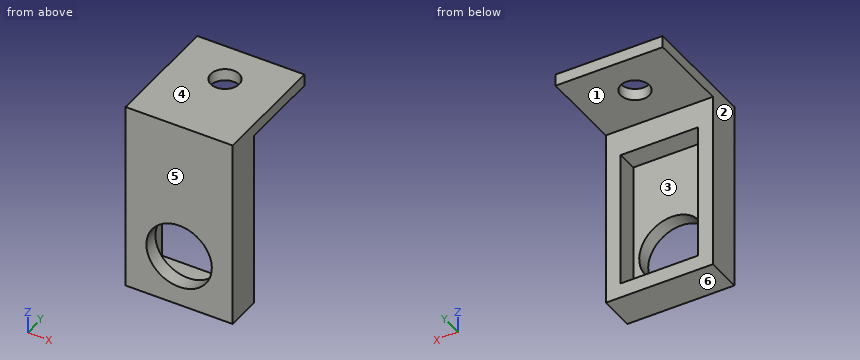
from build123d import *

# Parameters (mm, degrees)
SKETCH1_W           = 18
SKETCH1_H           = 32
BOSS_EXTRUDE1_DEPTH = 6
SKETCH2_W           = 13
SKETCH2_H           = 23
CUT_EXTRUDE1_DEPTH  = 3.5
SKETCH3_R           = 5.5
CUT_EXTRUDE2_DEPTH  = 37.881567212
SKETCH4_W           = 18
SKETCH4_H           = 2
BOSS_EXTRUDE2_DEPTH = 14
SKETCH5_R           = 2.4
CUT_EXTRUDE3_DEPTH  = 41.298883359


with BuildPart() as part:
    # Sketch1 → Boss-Extrude1 (new body)
    with BuildSketch(Plane(origin=(0, 0, 0), x_dir=(1, 0, 0), z_dir=(0, 1, 0))):
        with Locations((9, 16)):
            Rectangle(SKETCH1_W, SKETCH1_H)
    extrude(amount=BOSS_EXTRUDE1_DEPTH)

    # Sketch2 → Cut-Extrude1 (cut)
    with BuildSketch(Plane(origin=(0, 6, 0), x_dir=(1, 0, 0), z_dir=(0, 1, 0))):
        with Locations((9, 18)):
            Rectangle(SKETCH2_W, SKETCH2_H)
    extrude(amount=-CUT_EXTRUDE1_DEPTH, mode=Mode.SUBTRACT)

    # Sketch3 → Cut-Extrude2 (cut, through all)
    with BuildSketch(Plane(origin=(0, 2.5, 0), x_dir=(1, 0, 0), z_dir=(0, 1, 0))):
        with Locations(Location((9.000820155, 23.3, 0), (0, 0, 270))):
            Circle(SKETCH3_R)
    extrude(amount=-CUT_EXTRUDE2_DEPTH, mode=Mode.SUBTRACT)

    # Sketch4 → Boss-Extrude2 (add)
    with BuildSketch(Plane(origin=(0, 6, 0), x_dir=(1, 0, 0), z_dir=(0, 1, 0))):
        with Locations((9, 1)):
            Rectangle(SKETCH4_W, SKETCH4_H)
    extrude(amount=BOSS_EXTRUDE2_DEPTH)

    # Sketch5 → Cut-Extrude3 (cut, through all)
    with BuildSketch(Plane(origin=(0, 0, -2), x_dir=(-1, 0, 0), z_dir=(0, 0, -1))):
        with Locations((-8.774181154, 13.15523395)):
            Circle(SKETCH5_R)
    extrude(amount=-CUT_EXTRUDE3_DEPTH, mode=Mode.SUBTRACT)


solid = part.part
The model under review builds one solid part; all positions refer to its coordinate system, in mm. Face numbers are marked on the shaded views. A direction names the side the tool comes from. Round coordinates to 2 decimals unless told otherwise and drop trailing zeros. Write each loop counter-clockwise with the first axis right and the second up, starting at its lowest first coordinate (ties: lowest second). Pieces come first, ordered by that corner, then holes. Notation, with made-up numbers: (19.25, -18.75) - (64.25, -18.75) arc R31 cw to (64.25, 7.25) - close; hole circle Ø9 at (41, 78.25). An arc over 180 degrees is marked (long way). One line per item, written item: value. Start each with the question number.
1. Consider section D-D on z = -19. Write out the cut boundary in (x, y), and give its area (3 significant figures).
2. Consider section A-A on z = -23.3. Write out the cut boundary in (x, y).
3. Clearance check with flat-ended pins moving along their axes: P1, Ø3, axis at y = 9.5, z = -4, coming from the -X side; P2, Ø4, axis at x = 9, z = -13, coming from the +Y side; P3, Ø2, axis at x = 5, y = 13.5, coming from the -Z side. State where each tip first meets the part, or that it passes through.
4. The part is to be moulded in two halves that separate along Z. For the marked faces 3, 4, 5 and 6, say which applies: released by +Z, released by -Z, zero draft, split by the parting line, or undercut.
5. To check wall thickness, follow L1, parallel to X at y = 0.7, z = -23.3; L2, parallel to X at y = 5, z = -28; L3, parallel to Z at x = 13.75, y = 18.5. State the ranges of each line that lie inside material, in increasing order. Write a range as from..to.
6. Consider section C-C on x = 4. Write out the cut boundary in (y, z), and give its area (3 significant figures).
7. Consider section B-B on y = 4.75. Write out the cut boundary in (x, z).
8. Machinability: for the marked faces 1 and 2, which of the approach directions +Z, -Z, +X, -X, +Y, -Y give a long, thin tool a straight path to every point of the face, cutting with its end or side? Answer none if there is none.
Checks:
1. outline: (0, 0) - (5.57, 0) - (5.57, 2.5) - (2.5, 2.5) - (2.5, 6) - (0, 6) - close; (12.43, 0) - (18, 0) - (18, 6) - (15.5, 6) - (15.5, 2.5) - (12.43, 2.5) - close
1. area: 45.4 mm^2
2. outline: (0, 0) - (3.5, 0) - (3.5, 2.5) - (2.5, 2.5) - (2.5, 6) - (0, 6) - close; (14.5, 0) - (18, 0) - (18, 6) - (15.5, 6) - (15.5, 2.5) - (14.5, 2.5) - close
3. P1: passes through
3. P2: stops at y = 2.5
3. P3: stops at z = -2
4. face 3: undercut
4. face 4: released by +Z
4. face 5: zero draft
4. face 6: released by -Z
5. L1: x = 0..3.5, 14.5..18
5. L2: x = 0..2.5, 15.5..18
5. L3: z = -2..0
6. outline: (0, -32) - (6, -32) - (6, -29.5) - (2.5, -29.5) - (2.5, -25.59) - (0, -25.59) - close; (0, -21.01) - (2.5, -21.01) - (2.5, -6.5) - (6, -6.5) - (6, -2) - (20, -2) - (20, 0) - (0, 0) - close
6. area: 128 mm^2
7. outline: (0, -32) - (18, -32) - (18, 0) - (0, 0) - close; hole (2.5, -29.5) - (15.5, -29.5) - (15.5, -6.5) - (2.5, -6.5) - close
8. face 1: -Z, +X, -X, +Y
8. face 2: +Z, -Z, -X, +Y, -Y
